Source: CAD feature listing. Evaluate the final solid. Frame: model axes, mm. Round coordinates to 2 decimals unless told otherwise and drop trailing zeros. Loops run counter-clockwise (first coordinate to the right, second up) from the corner with the lowest first, then second, coordinate; pieces in that order, holes last. Notation, with made-up numbers: (-15, -23.75) -> (20, -23.75) arc R21 cw to (20, 1.25) -> close; hole circle Ø10 at (4.25, 9). An arc over 180 degrees is marked (long way). Put each result on its own line as item: value. Start each with the question number.
1. Cut plane A-A (z = 0). Return the cut outline in (x, y).
2. Cut plane B-B (y = 1.3). Return the cut outline in (x, z), then the cut area to 3 significant figures.
3. Draft query along Z for faces 1 (the cylindrical face through (-2.93, 0.92, 0.65)), 2 (the flat face through (-5, 3, 0)), 3 (the cylindrical face through (4.22, 2.24, -4.61)). Return one class per face: pulls with the +Z half, pulls with the -Z half, needs draft (parallel to the pull), parting line crosses it, or undercut.
4. Contact query for a flat-ended pin moving along its axis: pin 1 (1.5 mm diameter, centred on x = 4, y = 1, fed in from +Z). Output: stop coordinate, or through.
5. Material intervals for L1, parallel to X at y = 0.95, z = 0; L2, parallel to X at y = 1.9, z = 0; L3, parallel to Z at x = -2.75, y = 1, sorted ascending.
```python
from build123d import *

# Parameters (mm, degrees)
SKETCH_1_R               = 6.5
EXTRUDE_1_DEPTH          = 1.5
FILLET_1_R               = 1
SKETCH_2_R               = 6.25
EXTRUDE_2_DEPTH          = 1.5
CUT_EXTRUDE_1_DEPTH      = 10.66953987
CUT_EXTRUDE_1_DEPTH_BACK = 10.66953987
SKETCH_4_R               = 3
CUT_EXTRUDE_2_DEPTH      = 10.669539901


with BuildPart() as part:
    # 草图1 → 凸台-拉伸1 (new body)
    with BuildSketch(Plane(origin=(0, 0, 0), x_dir=(1, 0, 0), z_dir=(0, 1, 0))):
        with Locations(Location((0, 0, 0), (0, 0, 270))):
            Circle(SKETCH_1_R)
    extrude(amount=EXTRUDE_1_DEPTH)

    # 圆角1
    fillet_1_edges = [part.edges().sort_by_distance(p)[0] for p in [
        (0, 0, -6.5),
    ]]
    fillet(fillet_1_edges, radius=FILLET_1_R)

    # 草图2 → 凸台-拉伸2 (add)
    with BuildSketch(Plane(origin=(0, 1.5, 0), x_dir=(1, 0, 0), z_dir=(0, 1, 0))):
        with Locations(Location((0, 0, 0), (0, 0, 270))):
            Circle(SKETCH_2_R)
    extrude(amount=EXTRUDE_2_DEPTH)

    # 草图3 → 切除-拉伸1 (cut, two sides: drawn at the far end of the back side and taken through both)
    with BuildSketch(Plane.XY.offset(-CUT_EXTRUDE_1_DEPTH_BACK)):
        with BuildLine():
            ThreePointArc((-4, 3), (-2.096194346, 2.065792605), (0, 1.744562647))
            Line((0, 1.744562647), (0, 3))
            Line((0, 3), (-4, 3))
        make_face()
        with BuildLine():
            Line((0, 3), (0, 1.744562647))
            ThreePointArc((0, 1.744562647), (2.096194346, 2.065792605), (4, 3))
            Line((4, 3), (0, 3))
        make_face()
    extrude(amount=CUT_EXTRUDE_1_DEPTH + CUT_EXTRUDE_1_DEPTH_BACK, mode=Mode.SUBTRACT)

    # 草图4 → 切除-拉伸2 (cut, through all)
    with BuildSketch(Plane.XZ):
        with Locations(Location((0, 0, 0), (0, 0, 270))):
            Circle(SKETCH_4_R)
    extrude(amount=-CUT_EXTRUDE_2_DEPTH, mode=Mode.SUBTRACT)


solid = part.part
```
Solution:
1. outline: (-6.5, 1) arc R1 ccw to (-5.5, 0) -> (-3, 0) -> (-3, 2.42) arc R7 cw to (-4, 3) -> (-6.25, 3) -> (-6.25, 1.5) -> (-6.5, 1.5) -> close; (3, 0) -> (5.5, 0) arc R1 ccw to (6.5, 1) -> (6.5, 1.5) -> (6.25, 1.5) -> (6.25, 3) -> (4, 3) arc R7 cw to (3, 2.42) -> close
2. outline: circle Ø13 at (0, 0); hole circle Ø6 at (0, 0)
2. area: 104 mm^2
3. face 1: undercut
3. face 2: needs draft
3. face 3: parting line crosses it
4. pin 1: stops at z = 5.63
5. L1: x = -6.5 to -3, 3 to 6.5
5. L2: x = -6.25 to -3, 3 to 6.25
5. L3: z = -5.89 to -1.2, 1.2 to 5.89
